Model file for the job. Use its own axes, mm. Round coordinates to 2 decimals unless told otherwise and drop trailing zeros. Order: outer loops, then holes, each group sorted by start corner. A loop starts at its lowest first (then second) coordinate and runs counter-clockwise, first axis right, second up. Notation, with made-up numbers: (27, 36) - (42, 36) arc R21 cw to (42, 57) - close; hole circle Ø7 at (-30.75, -27). An arc over 180 degrees is marked (long way). Use one line per item in the form item = value.
from build123d import *

# Parameters (mm, degrees)
SKETCH1_W           = 43
SKETCH1_H           = 55
BOSS_EXTRUDE1_DEPTH = 3
SKETCH2_W           = 3
SKETCH2_H           = 27.5
CUT_EXTRUDE1_DEPTH  = 10
SKETCH3_R           = 1.1
SKETCH3_W           = 12.2
SKETCH3_H           = 22.5
CUT_EXTRUDE2_DEPTH  = 10


with BuildPart() as part:
    # Sketch1 → Boss-Extrude1 (new body)
    with BuildSketch(Plane(origin=(0, 0, 0), x_dir=(1, 0, 0), z_dir=(0, 1, 0))):
        Rectangle(SKETCH1_W, SKETCH1_H)
    extrude(amount=BOSS_EXTRUDE1_DEPTH)

    # Sketch2 → Cut-Extrude1 (cut)
    with BuildSketch(Plane(origin=(0, 3, 0), x_dir=(1, 0, 0), z_dir=(0, 1, 0))):
        with Locations((0, -13.75)):
            Rectangle(SKETCH2_W, SKETCH2_H)
    extrude(amount=-CUT_EXTRUDE1_DEPTH, mode=Mode.SUBTRACT)

    # Sketch3 → Cut-Extrude2 (cut)
    with BuildSketch(Plane.XZ):
        with Locations(Location((12.9, -25.35, 0), (0, 0, 270))):
            Circle(SKETCH3_R)
        with Locations(Location((12.9, 2.45, 0), (0, 0, 270))):
            Circle(SKETCH3_R)
        with Locations(Location((-12.9, -25.35, 0), (0, 0, 270))):
            Circle(SKETCH3_R)
        with Locations(Location((-12.9, 2.45, 0), (0, 0, 270))):
            Circle(SKETCH3_R)
        with Locations((12.9, -11.45)):
            Rectangle(SKETCH3_W, SKETCH3_H)
        with Locations((-12.9, -11.45)):
            Rectangle(SKETCH3_W, SKETCH3_H)
    extrude(amount=-CUT_EXTRUDE2_DEPTH, mode=Mode.SUBTRACT)


solid = part.part
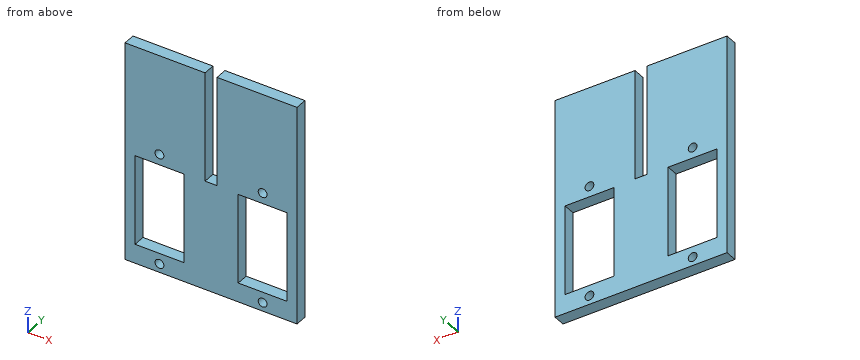
(1) Probe probe 1 along X at (y, z) = (1.75, 2.45); probe 2 along X at (y, z) = (2.6, -9.5); probe 3 along X at (y, z) = (1.85, -25.35). List the from-to ranges inside material, lowest first. Write a range as [from, to].
Report:
probe_1 = [-21.5, -14], [-11.8, -1.5], [1.5, 11.8], [14, 21.5]
probe_2 = [-21.5, -19], [-6.8, 6.8], [19, 21.5]
probe_3 = [-21.5, -14], [-11.8, 11.8], [14, 21.5]
(2) Slice it at A-A on x = 16.5. Give the cut face in (y, z).
Report:
outline = (0, -27.5) - (3, -27.5) - (3, -22.7) - (0, -22.7) - close; (0, -0.2) - (3, -0.2) - (3, 27.5) - (0, 27.5) - close
(3) Slice it at B-B on y = 2.05. Give the cut face in (x, z), then the cut area to 3 significant figures.
Report:
outline = (-21.5, -27.5) - (21.5, -27.5) - (21.5, 27.5) - (1.5, 27.5) - (1.5, 0) - (-1.5, 0) - (-1.5, 27.5) - (-21.5, 27.5) - close; hole (-19, -22.7) - (-6.8, -22.7) - (-6.8, -0.2) - (-19, -0.2) - close; hole circle Ø2.2 at (-12.9, -25.35); hole circle Ø2.2 at (-12.9, 2.45); hole (6.8, -22.7) - (19, -22.7) - (19, -0.2) - (6.8, -0.2) - close; hole circle Ø2.2 at (12.9, -25.35); hole circle Ø2.2 at (12.9, 2.45)
area = 1,720 mm2
(4) Pin check, flat tip, straight feed: pin 1 (2 mm diameter, centred on x = -12.9, z = -25.35, fed in from -Y). Stop position of the tip, or through.
Report:
pin_1 = through
(5) Slice it at C-C on z = -25.35. Give the cut face in (x, y), then the cut area to 3 significant figures.
Report:
outline = (-21.5, 0) - (-14, 0) - (-14, 3) - (-21.5, 3) - close; (-11.8, 0) - (11.8, 0) - (11.8, 3) - (-11.8, 3) - close; (14, 0) - (21.5, 0) - (21.5, 3) - (14, 3) - close
area = 116 mm2
(6) Slice it at D-D on z = 23. Give the cut face in (x, y), then the cut area to 3 significant figures.
Report:
outline = (-21.5, 0) - (-1.5, 0) - (-1.5, 3) - (-21.5, 3) - close; (1.5, 0) - (21.5, 0) - (21.5, 3) - (1.5, 3) - close
area = 120 mm2
